```python
from build123d import *

# Parameters (mm, degrees)
SKETCH1_W                               = 180
SKETCH1_H                               = 180
BOSS_EXTRUDE1_DEPTH                     = 10
SKETCH2_R                               = 70
BOSS_EXTRUDE2_DEPTH                     = 80
SKETCH3_W                               = 80
SKETCH3_H                               = 40
BOSS_EXTRUDE3_DEPTH                     = 90
SKETCH4_R                               = 65
CUT_EXTRUDE1_DEPTH                      = 3
CBORE_FOR_M6_HEX_HEAD_BOLT1_D           = 6.6
CBORE_FOR_M6_HEX_HEAD_BOLT1_CBORE_D     = 14.55
CBORE_FOR_M6_HEX_HEAD_BOLT1_CBORE_DEPTH = 4.38
FILLET1_R                               = 10


with BuildPart() as part:
    # Sketch1 → Boss-Extrude1 (new body)
    with BuildSketch(Plane(origin=(0, 0, 0), x_dir=(1, 0, 0), z_dir=(0, 1, 0))):
        with Locations((-49.591836735, -5.510204082)):
            Rectangle(SKETCH1_W, SKETCH1_H)
    extrude(amount=BOSS_EXTRUDE1_DEPTH)

    # Sketch2 → Boss-Extrude2 (add)
    with BuildSketch(Plane(origin=(0, 10, 0), x_dir=(1, 0, 0), z_dir=(0, 1, 0))):
        with Locations((-57.006666854, 0)):
            Circle(SKETCH2_R)
    extrude(amount=BOSS_EXTRUDE2_DEPTH)

    # Sketch3 → Boss-Extrude3 (add)
    with BuildSketch(Plane.XY):
        with Locations((-49.893940427, 49.288531055)):
            Rectangle(SKETCH3_W, SKETCH3_H)
    extrude(amount=BOSS_EXTRUDE3_DEPTH)

    # Sketch4 → Cut-Extrude1 (cut)
    with BuildSketch(Plane(origin=(0, 90, 0), x_dir=(1, 0, 0), z_dir=(0, 1, 0))):
        with Locations((-57.006666854, 0)):
            Circle(SKETCH4_R)
    extrude(amount=-CUT_EXTRUDE1_DEPTH, mode=Mode.SUBTRACT)

    # CBORE for M6 Hex Head Bolt1 (through all)
    with Locations(Plane(origin=(0, 10, 0), x_dir=(1, 0, 0), z_dir=(0, 1, 0))):
        with Locations((-121.727687168, 66.314718067), (18.854420034, 66.314718067), (18.854420034, -76.9115667), (-121.727687168, -79.996440525)):
            CounterBoreHole(CBORE_FOR_M6_HEX_HEAD_BOLT1_D / 2, CBORE_FOR_M6_HEX_HEAD_BOLT1_CBORE_D / 2, CBORE_FOR_M6_HEX_HEAD_BOLT1_CBORE_DEPTH)

    # Fillet1
    fillet1_edges = [part.edges().sort_by_distance(p)[0] for p in [
        (-89.893940427, 49.288531055, 90),
        (-9.893940427, 49.288531055, 90),
        (-139.591836735, 5, -84.489795918),
        (40.408163265, 5, -84.489795918),
        (40.408163265, 5, 95.510204082),
        (-139.591836735, 5, 95.510204082),
    ]]
    fillet(fillet1_edges, radius=FILLET1_R)


solid = part.part
```
Build history of the part. All positions in model axes, mm. A direction names the side the tool comes from. Round coordinates to 2 decimals unless told otherwise and drop trailing zeros. Write each loop counter-clockwise with the first axis right and the second up, starting at its lowest first coordinate (ties: lowest second). Pieces come first, ordered by that corner, then holes. Notation, with made-up numbers: (-12, -4.75) - (8, -4.75) arc R28 ccw to (8, 30.25) - close; hole circle Ø5 at (63.5, 42.5). An arc over 180 degrees is marked (long way). Write each question's results on one line, items separated by ' | '. Start each with the question number.
Item 1: Wall check: L1, parallel to Y at x = 1, z = 47.5; L2, parallel to Y at x = -4.5, z = -29; L3, parallel to Z at x = -64, y = 77. Give the ranges that are in metal, low to high. Write a range as [from, to].
Item 2: Drop flat-ended pins along their axis: P1, Ø16, axis at x = -119.5, z = 79.5, coming from the +Y side; P2, Ø4, axis at x = -56, y = 45.5, coming from the +Z side; P3, Ø2, axis at y = 35.5, z = -38.5, coming from the +X side; P4, Ø4, axis at x = 18.85, z = 76.91, coming from the +Y side. Give the stop position or say it passes through.
Item 3: Saw through at A-A (z = 0). Write the cut outline in (x, y), and give its area (3 significant figures).
Item 4: Saw through at B-B (x = -5). Write the cut outline in (y, z), and give its area (3 significant figures).
Item 5: Which spindle directions (+Z, -Z, +X, -X, +Y, -Y) get a long thin tool onto all of the face, cutting with end or side? Do faces 1 (the face through (-9.894, 49, 66)), 2 (the face through (-139.592, 5, 7)), 3 (the face through (17.277, 7.841, 84.014)). Say none if no direction does.
Item 6: Mould opens along X. For faces 4 (the face through (-50, 50, 90)), 5 (the face through (20.4, 5.62, 80)), 6 (the face through (-89.894, 49, 71)), 7 (the face through (-115.007, 7.841, -63.528)) say: pulls with the +X half, pulls with the -X half, needs draft (parallel to the pull), parting line crosses it, or undercut.
Item 7: Saw through at D-D (x = -26). Write the cut outline in (y, z), and give its area (3 significant figures).
Item 8: Saw through at C-C (y = 41). Write the cut outline in (x, z), and give its area (3 significant figures).
Results are:
1) L1: y = [0, 10] | L2: y = [0, 87] | L3: z = [-69.65, 69.65]
2) P1: stops at y = 10 | P2: stops at z = 90 | P3: stops at x = 2.1 | P4: passes through
3) outline: (-139.59, 0) - (40.41, 0) - (40.41, 10) - (12.99, 10) - (12.99, 90) - (7.99, 90) - (7.99, 87) - (-122.01, 87) - (-122.01, 90) - (-127.01, 90) - (-127.01, 10) - (-139.59, 10) - close | area: 12,600 mm²
4) outline: (0, -84.49) - (10, -84.49) - (10, -46.85) - (90, -46.85) - (90, -38.99) - (87, -38.99) - (87, 38.99) - (90, 38.99) - (90, 46.85) - (10, 46.85) - (10, 95.51) - (0, 95.51) - close | area: 9,060 mm²
5) face 1: +Z, +X, +Y | face 2: +Z, -Z, -X, +Y, -Y | face 3: +Y
6) face 4: needs draft | face 5: undercut | face 6: pulls with the -X half | face 7: undercut
7) outline: (0, -84.49) - (10, -84.49) - (10, -62.76) - (90, -62.76) - (90, -57.13) - (87, -57.13) - (87, 57.13) - (90, 57.13) - (90, 62.76) - (69.29, 62.76) - (69.29, 90) - (29.29, 90) - (29.29, 62.76) - (10, 62.76) - (10, 95.51) - (0, 95.51) - close | area: 12,600 mm²
8) outline: (-89.89, 61.79) arc R70 ccw (long way) to (-9.89, 51.77) - (-9.89, 80) arc R10 ccw to (-19.89, 90) - (-79.89, 90) arc R10 ccw to (-89.89, 80) - close | area: 17,300 mm²
